For this review, take the finished solid that the model builds, in its own axes (mm). Give positions to 0.01 mm unless a question says otherwise; leave off trailing zeros. Order: outer loops, then holes, each group sorted by start corner. A loop starts at its lowest first (then second) coordinate and runs counter-clockwise, first axis right, second up. Notation, with made-up numbers: M 39.25,-18 L 50.25,-18 A17 cw 50.25,-2 Z; hole C -25,18 d9. An arc over 180 degrees is marked long. Use CSV: the item, a comma, the result in double quotes. Start each with the question number.
(1) Clearance check with flat-ended pins moving along their axes: P1, Ø5.5, axis at x = 136, y = 140, coming from the +Z side; P2, Ø2.5, axis at x = -136, y = 40, coming from the +Z side; P3, Ø1.6, axis at y = -144, z = 5.5, coming from the +X side; P4, Ø4, axis at x = 136, y = -85, coming from the -Z side. State where each tip first meets the part, or that it passes through.
(2) Consider section C-C (z = 1.05). Give the number of separate pieces and of enclosed holes in the cut face, and give its area (3 significant figures).
(3) Consider section B-B (x = -58.5). Write out the cut boundary in (y, z), and give its area (3 significant figures).
(4) Consider section A-A (y = 27.5). Write out the cut boundary in (x, z).
(5) Wall thickness on L1, parallel to X at y = 90, z = 2.55; L2, parallel to Y at x = 6, z = 2.6; L3, parallel to X at y = 50.5, z = 2.5: over which ranges is each line inside the solid? List them lowest first. Write a range as from..to.
```python
from build123d import *

# Parameters (mm, degrees)
F0_W     = 324
F0_H     = 300
F1_DEPTH = 6
F2_R     = 10
F3_W     = 22
F3_H     = 2
F4_DEPTH = 300
F6_D     = 3.3
F6_DEPTH = 14.1
F6_TIP   = 0.9914200214
F7_R     = 10


with BuildPart() as f1:
    # F0 (on Top) → F1 (new body)
    with BuildSketch(Plane.XY):
        Rectangle(F0_W, F0_H)
        Polygon((-130, 0), (-130, 130), (130, 130), (130, 0), (130, -130), (-130, -130), align=None, mode=Mode.SUBTRACT)
    extrude(amount=F1_DEPTH)

    # F2
    f2_edges = [f1.edges().sort_by_distance(p)[0] for p in [
        (130, 130, 3),
        (-130, 130, 3),
        (-130, -130, 3),
        (130, -130, 3),
    ]]
    fillet(f2_edges, radius=F2_R)

    # F3 (on face) → F4 (cut)
    with BuildSketch(Plane.XZ.offset(150)):
        with Locations((-131, 5)):
            Rectangle(F3_W, F3_H)
        with Locations((131, 5)):
            Rectangle(F3_W, F3_H)
    extrude(amount=-F4_DEPTH, mode=Mode.SUBTRACT)

    # F6
    with Locations(Plane.XY.offset(4)):
        with Locations((-136, 140), (-136, 90), (-136, -135), (136, -135), (136, 90), (136, 140), (136, -85), (-136, -85), (-136, 40), (-136, -35), (136, -35), (136, 40)):
            Hole(F6_D / 2, depth=F6_DEPTH)
            with Locations((0, 0, -(F6_DEPTH + F6_TIP / 2))):  # 118° drill point
                Cone(0, F6_D / 2, F6_TIP, mode=Mode.SUBTRACT)

    # F7
    f7_edges = [f1.edges().sort_by_distance(p)[0] for p in [
        (162, -150, 3),
        (162, 150, 3),
        (-162, -150, 3),
        (-162, 150, 3),
    ]]
    fillet(f7_edges, radius=F7_R)


solid = f1.part
```
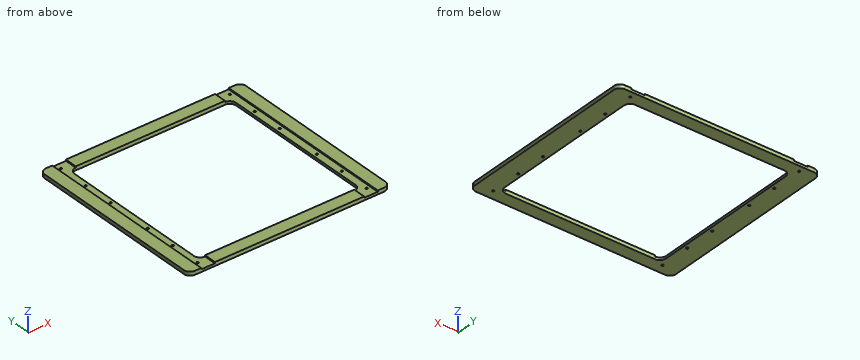
Check result:
1,P1,"stops at z = 4"
1,P2,"passes through"
1,P3,"stops at x = 161.47"
1,P4,"stops at z = 0"
2,separate pieces,"1"
2,enclosed holes,"13"
2,area,"29,500 mm^2"
3,outline,"M -150,0 L -130,0 L -130,6 L -150,6 Z; M 130,0 L 150,0 L 150,6 L 130,6 Z"
3,area,"240 mm^2"
4,outline,"M -162,0 L -130,0 L -130,4 L -142,4 L -142,6 L -162,6 Z; M 130,0 L 162,0 L 162,6 L 142,6 L 142,4 L 130,4 Z"
5,L1,"x = -162..-137.65, -134.35..-130, 130..134.35, 137.65..162"
5,L2,"y = -150..-130, 130..150"
5,L3,"x = -162..-130, 130..162"
